Check sheet for the modelled part. Datum: model origin and axes. Units: mm. A direction names the side the tool comes from. Give positions to 0.01 mm unless a question says otherwise; leave off trailing zeros. Write each loop counter-clockwise with the first axis right and the second up, starting at its lowest first coordinate (ties: lowest second). Pieces come first, ordered by that corner, then holes.
from build123d import *

# Parameters (mm, degrees)
F0_R     = 11
F0_R_2   = 5
F1_DEPTH = 1.5
F0_R_3   = 4
F2_DEPTH = 2
F3_DEPTH = 5
F4_R     = 1


with BuildPart() as f1:
    # F0 (on Top) → F1 (new body)
    with BuildSketch(Plane.XY):
        Circle(F0_R)
        Circle(F0_R_2, mode=Mode.SUBTRACT)
    extrude(amount=F1_DEPTH)

    # F0 (on Top) → F2 (join)
    with BuildSketch(Plane.XY):
        Circle(F0_R_2)
        Circle(F0_R_3, mode=Mode.SUBTRACT)
    extrude(amount=F2_DEPTH)

    # F0 (on Top) → F3 (join)
    with BuildSketch(Plane.XY):
        Circle(F0_R_3)
    extrude(amount=F3_DEPTH)

    # F4
    f4_edges = [f1.edges().sort_by_distance(p)[0] for p in [
        (-11, 0, 0),
    ]]
    fillet(f4_edges, radius=F4_R)


solid = f1.part
1) Sectioned sample at C-C on z = 2.9. Record the boundary of the cut face in (x, y), then the cut area to 3 significant figures.
2) Sectioned sample at D-D on z = 0.5. Record the boundary of the cut face in (x, y).
3) Gauge pin test, flat ends, axial feed: pin 1 (1 mm diameter, centred on y = 5, z = 1, fed in from +X); pin 2 (2 mm diameter, centred on y = 4, z = 0.5, fed in from -X). Record the tip position at first contact, or that the pin passes through.
4) Scan lines: L1, parallel to Z at x = -5, y = 1.5; L2, parallel to Z at x = 1.25, y = 4.25; L3, parallel to X at y = -7, z = 0.3. Record each from-to range of solid material in increasing order.
5) Access from +Z, -Z, +X, -X, +Y, -Y to the whole of each face (thin tool, end or side, straight path). Record for faces 1 (the cylindrical face through (-1.08, -4.88, 1.75)), 2 (the flat face through (0, 0, 0)).
6) Sectioned sample at A-A on x = 0. Record the boundary of the cut face in (y, z).
Answers below:
1. outline: circle Ø8 at (0, 0)
1. area: 50.3 mm2
2. outline: circle Ø21.73 at (0, 0)
3. pin 1: stops at x = 10.04
3. pin 2: stops at x = -10.55
4. L1: z = 0 to 1.5
4. L2: z = 0 to 2
4. L3: x = -8.11 to 8.11
5. face 1: +Z
5. face 2: -Z, +X, -X, +Y, -Y
6. outline: (-11, 1) arc R1 ccw to (-10, 0) - (10, 0) arc R1 ccw to (11, 1) - (11, 1.5) - (5, 1.5) - (5, 2) - (4, 2) - (4, 5) - (-4, 5) - (-4, 2) - (-5, 2) - (-5, 1.5) - (-11, 1.5) - close
